from build123d import *

# Parameters (mm, degrees)
SKETCH1_W           = 177.8
SKETCH1_H           = 139.7
BOSS_EXTRUDE1_DEPTH = 12.7
CUT_EXTRUDE1_DEPTH  = 9.525


with BuildPart() as part:
    # Sketch1 → Boss-Extrude1 (new body)
    with BuildSketch(Plane.XY):
        Rectangle(SKETCH1_W, SKETCH1_H)
    extrude(amount=BOSS_EXTRUDE1_DEPTH)

    # Sketch2 → Cut-Extrude1 (cut)
    with BuildSketch(Plane.XY.offset(12.7)):
        with BuildLine():
            Line((-65.0875, 63.5), (65.0875, 63.5))
            ThreePointArc((65.0875, 63.5), (68.455096045, 62.105096045), (69.85, 58.7375))
            Line((69.85, 58.7375), (69.85, 42.8625))
            ThreePointArc((69.85, 42.8625), (71.244903955, 39.494903955), (74.6125, 38.1))
            Line((74.6125, 38.1), (77.7875, 38.1))
            ThreePointArc((77.7875, 38.1), (81.155096045, 36.705096045), (82.55, 33.3375))
            Line((82.55, 33.3375), (82.55, 4.7625))
            ThreePointArc((82.55, 4.7625), (81.155096045, 1.394903955), (77.7875, 0))
            Line((77.7875, 0), (42.8625, 0))
            ThreePointArc((42.8625, 0), (39.494903955, -1.394903955), (38.1, -4.7625))
            Line((38.1, -4.7625), (38.1, -20.6375))
            ThreePointArc((38.1, -20.6375), (36.705096045, -24.005096045), (33.3375, -25.4))
            Line((33.3375, -25.4), (23.8125, -25.4))
            ThreePointArc((23.8125, -25.4), (20.444903955, -26.794903955), (19.05, -30.1625))
            Line((19.05, -30.1625), (19.05, -46.0375))
            ThreePointArc((19.05, -46.0375), (17.655096045, -49.405096045), (14.2875, -50.8))
            Line((14.2875, -50.8), (-65.0875, -50.8))
            ThreePointArc((-65.0875, -50.8), (-68.455096045, -49.405096045), (-69.85, -46.0375))
            Line((-69.85, -46.0375), (-69.85, -30.1625))
            ThreePointArc((-69.85, -30.1625), (-68.455096045, -26.794903955), (-65.0875, -25.4))
            Line((-65.0875, -25.4), (1.5875, -25.4))
            ThreePointArc((1.5875, -25.4), (4.955096045, -24.005096045), (6.35, -20.6375))
            Line((6.35, -20.6375), (6.35, 0))
            Line((6.35, 0), (6.35, 33.3375))
            ThreePointArc((6.35, 33.3375), (4.955096045, 36.705096045), (1.5875, 38.1))
            Line((1.5875, 38.1), (-58.7375, 38.1))
            ThreePointArc((-58.7375, 38.1), (-62.105096045, 36.705096045), (-63.5, 33.3375))
            Line((-63.5, 33.3375), (-63.5, 4.7625))
            ThreePointArc((-63.5, 4.7625), (-64.894903955, 1.394903955), (-68.2625, 0))
            Line((-68.2625, 0), (-77.7875, 0))
            ThreePointArc((-77.7875, 0), (-81.155096045, 1.394903955), (-82.55, 4.7625))
            Line((-82.55, 4.7625), (-82.55, 33.3375))
            ThreePointArc((-82.55, 33.3375), (-81.155096045, 36.705096045), (-77.7875, 38.1))
            Line((-77.7875, 38.1), (-74.6125, 38.1))
            ThreePointArc((-74.6125, 38.1), (-71.244903955, 39.494903955), (-69.85, 42.8625))
            Line((-69.85, 42.8625), (-69.85, 58.7375))
            ThreePointArc((-69.85, 58.7375), (-68.455096045, 62.105096045), (-65.0875, 63.5))
        make_face()
        with BuildLine():
            Line((42.8625, -25.4), (77.7875, -25.4))
            ThreePointArc((77.7875, -25.4), (81.155096045, -26.794903955), (82.55, -30.1625))
            Line((82.55, -30.1625), (82.55, -46.0375))
            ThreePointArc((82.55, -46.0375), (81.155096045, -49.405096045), (77.7875, -50.8))
            Line((77.7875, -50.8), (42.8625, -50.8))
            ThreePointArc((42.8625, -50.8), (39.494903955, -49.405096045), (38.1, -46.0375))
            Line((38.1, -46.0375), (38.1, -30.1625))
            ThreePointArc((38.1, -30.1625), (39.494903955, -26.794903955), (42.8625, -25.4))
        make_face()
    extrude(amount=-CUT_EXTRUDE1_DEPTH, mode=Mode.SUBTRACT)


solid = part.part
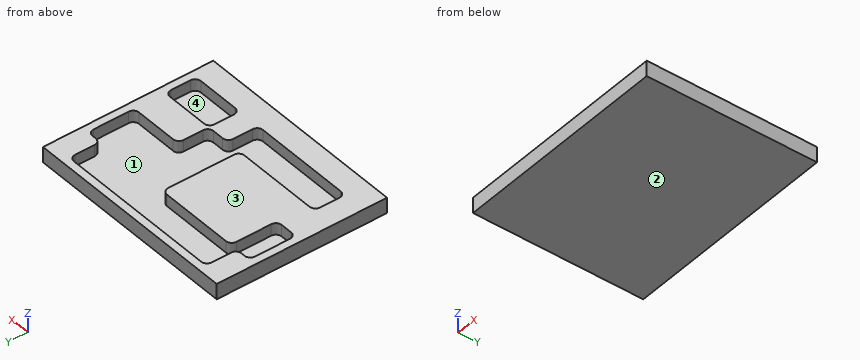
The listing builds one solid part. Answer for the finished solid, in the listing's coordinates (mm). Face numbers are marked on the shaded views. A direction names the side the tool comes from. Coordinates: 2 decimals unless noted, no trailing zeros. Write each loop counter-clockwise with the first axis right and the second up, starting at its lowest first coordinate (ties: lowest second). Pieces come first, ordered by that corner, then holes. Notation, with made-up numbers: (68.5, 61.25) - (105.5, 61.25) arc R18 ccw to (105.5, 88.25) - close; hole circle Ø3 at (57.25, 61). An arc over 180 degrees is marked (long way). Answer as CSV lines item,"result".
1. Find section B-B (y = 20.5). Give the vertices of the cut face in (x, z) (3 decimals).
Computed values:
outline,"(-88.9, 0) - (88.9, 0) - (88.9, 12.7) - (82.55, 12.7) - (82.55, 3.175) - (6.35, 3.175) - (6.35, 12.7) - (-63.5, 12.7) - (-63.5, 3.175) - (-82.55, 3.175) - (-82.55, 12.7) - (-88.9, 12.7) - close"
2. Determine the mould class of the marked faces 1 and 2 for opening direction Z: +Z half, -Z half, draft (parallel to the pull), parting line (faces both ways), or undercut.
Computed values:
face 1,"+Z half"
face 2,"-Z half"
3. A tool of negligible diameter and unlimited length cuts with its end or side. For the marked faces 3 and 4, from which of +Z, -Z, +X, -X, +Y, -Y can it reach the whole face along a straight path? Write none if from no direction.
Computed values:
face 3,"+Z, +X, -X, +Y, -Y"
face 4,"+Z"
4. Find section C-C (z = 7.25). Give the number of separate pieces and of enclosed holes in the cut face, plus the area to 3 significant figures.
Computed values:
separate pieces,"1"
enclosed holes,"2"
area,"13,500 mm²"
5. Straight lines are drawn through the part: line 1 (X direction, y = -30.5, z = 9.5); line 2 (Y direction, x = 51.5, z = 9.75); line 3 (X direction, y = 26, z = 8). For each, find the intervals that lie inside material, in ascending order. Write a range as [from, to].
Computed values:
line 1,"x = [-88.9, -69.85], [19.05, 38.1], [82.55, 88.9]"
line 2,"y = [-69.85, -50.8], [-25.4, 0], [63.5, 69.85]"
line 3,"x = [-88.9, -82.55], [-63.5, 6.35], [82.55, 88.9]"
6. Find section D-D (y = -17). Give the vertices of the cut face in (x, z) (3 decimals), plus the area to 3 significant figures.
Computed values:
outline,"(-88.9, 0) - (88.9, 0) - (88.9, 12.7) - (38.1, 12.7) - (38.1, 3.175) - (6.35, 3.175) - (6.35, 12.7) - (-88.9, 12.7) - close"
area,"1,960 mm²"
7. Find section A-A (x = 49.5). Give the vertices of the cut face in (y, z) (3 decimals).
Computed values:
outline,"(-69.85, 0) - (69.85, 0) - (69.85, 12.7) - (63.5, 12.7) - (63.5, 3.175) - (0, 3.175) - (0, 12.7) - (-25.4, 12.7) - (-25.4, 3.175) - (-50.8, 3.175) - (-50.8, 12.7) - (-69.85, 12.7) - close"
8. Given P1, Ø2, axis at x = -14, y = -38.5, coming from the +Z side (3 decimals), flat-ended and moving along its own axis, determine where the tip first touches the part or whether it passes through.
Computed values:
P1,"stops at z = 3.175"
